Build history of the part. All positions in model axes, mm. A direction names the side the tool comes from. Round coordinates to 2 decimals unless told otherwise and drop trailing zeros. Write each loop counter-clockwise with the first axis right and the second up, starting at its lowest first coordinate (ties: lowest second). Pieces come first, ordered by that corner, then holes. Notation, with made-up numbers: M 80,49 L 124,49 A21 ccw 124,72 Z; hole C 65.25,48.25 d5. An arc over 180 degrees is marked long. Write item = value, one per line. Start each with the question number.
Q1. Drop flat-ended pins along their axis: P1, Ø4, axis at y = -22.5, z = 5, coming from the -X side; P2, Ø10, axis at x = -8.5, y = 9.5, coming from the +Z side; P3, Ø1.5, axis at x = -44.5, z = 13, coming from the +Y side; P4, Ø2.5, axis at y = 24.5, z = 13, coming from the +X side. Give the stop position or say it passes through.
Q2. Band-saw the part on A-A on x = 51. Write the cut outline in (y, z), plus the area to 3 significant figures.
Q3. Pull direction Y, two halves, no side cores. Call faces 5 (the flat face through (0, 18, 0)), 6 (the flat face through (0, 33.092, 7)), 7 (the flat face through (0, 34.092, 13)): released by +Y, released by -Y, zero draft, split by the parting line, or undercut.
Q4. Probe L1, parallel to X at y = 24, z = 14; L2, parallel to Y at x = -74.5, z = 6.25; L3, parallel to Y at x = -62.5, z = 10.5. List the from-to ranges inside material, lowest first.
Q5. Band-saw the part on D-D on z = 12.25. Write the cut outline in (x, y).
Q6. Band-saw the part on B-B on y = -47. Write the cut outline in (x, z), plus the area to 3 significant figures.
Q7. Tool access for faces 1 (the flat face through (-83.74, -12, 13)), 2 (the flat face through (2, -54.908, 10)), 3 (the flat face through (1, -56, 5.762)), 4 (the flat face through (-82.74, -2, 9)): list every direction of +Z, -Z, +X, -X, +Y, -Y with a clear straight run to the whole face (end or side of a thin tool).
Q8. Band-saw the part on C-C on x = 16. Write the cut outline in (y, z), plus the area to 3 significant figures.
```python
from build123d import *

# Parameters (mm, degrees)
SKETCH_1_W               = 172
SKETCH_1_H               = 92
EXTRUDE_1_DEPTH          = 2
SKETCH_2_W               = 32
SKETCH_2_H               = 22
CUT_EXTRUDE_1_DEPTH      = 2
SKETCH_3_R               = 6.5
CUT_EXTRUDE_2_DEPTH      = 2
SKETCH_4_W               = 172
SKETCH_4_H               = 92
EXTRUDE_3_DEPTH          = 13
SKETCH_5_W               = 168
SKETCH_5_H               = 55.87
CUT_EXTRUDE_3_DEPTH      = 18
CUT_EXTRUDE_4_DEPTH      = 182.789670088
CUT_EXTRUDE_4_DEPTH_BACK = 172
FILLET_1_R               = 15
SKETCH_7_W               = 10
SKETCH_7_H               = 10
CUT_EXTRUDE_5_DEPTH      = 2
CUT_EXTRUDE_6_DEPTH      = 5
FILLET_2_R               = 2
FILLET_3_R               = 1.5


with BuildPart() as part:
    # 草图1 → 凸台-拉伸1 (new body)
    with BuildSketch(Plane.XY):
        with Locations((1.259970458, -10.907680945)):
            Rectangle(SKETCH_1_W, SKETCH_1_H)
    extrude(amount=EXTRUDE_1_DEPTH)

    # 草图2 → 切除-拉伸1 (cut)
    with BuildSketch(Plane(origin=(0, 0, 0), x_dir=(-1, 0, 0), z_dir=(0, 0, -1))):
        with Locations((-60.259970458, 22.092319055)):
            Rectangle(SKETCH_2_W, SKETCH_2_H)
    extrude(amount=-CUT_EXTRUDE_1_DEPTH, mode=Mode.SUBTRACT)

    # 草图3 → 切除-拉伸2 (cut)
    with BuildSketch(Plane(origin=(0, 0, 0), x_dir=(-1, 0, 0), z_dir=(0, 0, -1))):
        with Locations((54.740029542, 24.092319055)):
            Circle(SKETCH_3_R)
        with Locations((71.740029542, 25.092319055)):
            Circle(SKETCH_3_R)
    extrude(amount=-CUT_EXTRUDE_2_DEPTH, mode=Mode.SUBTRACT)

    # 草图4 → 凸台-拉伸3 (add)
    with BuildSketch(Plane.XY.offset(2)):
        with Locations((1.259970458, -10.907680945)):
            Rectangle(SKETCH_4_W, SKETCH_4_H)
        Polygon((-82.740029542, -54.907680945), (-82.740029542, 33.092319055), (44.259970458, 33.092319055), (76.259970458, 33.092319055), (85.259970458, 33.092319055), (85.259970458, -54.907680945), align=None, mode=Mode.SUBTRACT)
    extrude(amount=EXTRUDE_3_DEPTH)

    # 草图5 → 切除-拉伸3 (cut)
    with BuildSketch(Plane(origin=(0, 0, 0), x_dir=(-1, 0, 0), z_dir=(0, 0, -1))):
        with Locations((-1.259970458, -26.972680945)):
            Rectangle(SKETCH_5_W, SKETCH_5_H)
    extrude(amount=-CUT_EXTRUDE_3_DEPTH, mode=Mode.SUBTRACT)

    # 草图6 → 切除-拉伸4 (cut, two sides: drawn at the far end of the back side and taken through both)
    with BuildSketch(Plane(origin=(87.259970458, 0, 0), x_dir=(0, 0, -1), z_dir=(1, 0, 0)).offset(-CUT_EXTRUDE_4_DEPTH_BACK)):
        Polygon((84.64151075, 176.551763032), (0, 0.962319055), (-5.76238744, -10.991796575), (-5.76238744, -56.907680945), (-5.76238744, -251.832892702), (375.68654555, -332.33173887), (466.09044374, 96.052916865), align=None)
    extrude(amount=CUT_EXTRUDE_4_DEPTH + CUT_EXTRUDE_4_DEPTH_BACK, mode=Mode.SUBTRACT)

    # 圆角1
    fillet_1_edges = [part.edges().sort_by_distance(p)[0] for p in [
        (86.259970458, -10.991796575, 5.76238744),
        (-83.740029542, -10.991796575, 5.76238744),
    ]]
    fillet(fillet_1_edges, radius=FILLET_1_R)

    # 草图7 → 切除-拉伸5 (cut)
    with BuildSketch(Plane(origin=(87.259970458, 0, 0), x_dir=(0, 0, -1), z_dir=(1, 0, 0))):
        with Locations((-10, 12.092319055)):
            Rectangle(SKETCH_7_W, SKETCH_7_H)
    extrude(amount=-CUT_EXTRUDE_5_DEPTH, mode=Mode.SUBTRACT)

    # 草图8 → 切除-拉伸6 (cut)
    with BuildSketch(Plane.XY.offset(15)):
        Polygon((-83.740029542, -55.907680945), (-83.740029542, 34.092319055), (86.259970458, 34.092319055), (86.259970458, 17.092319055), (87.259970458, 17.092319055), (87.259970458, 35.092319055), (-84.740029542, 35.092319055), (-84.740029542, -56.907680945), (87.259970458, -56.907680945), (87.259970458, 7.092319055), (86.259970458, 7.092319055), (86.259970458, -55.907680945), align=None)
    extrude(amount=-CUT_EXTRUDE_6_DEPTH, mode=Mode.SUBTRACT)

    # 圆角2
    fillet_2_edges = [part.edges().sort_by_distance(p)[0] for p in [
        (76.259970458, 11.092319055, 1),
        (76.259970458, 33.092319055, 1),
        (44.259970458, 33.092319055, 1),
        (44.259970458, 11.092319055, 1),
    ]]
    fillet(fillet_2_edges, radius=FILLET_2_R)

    # 圆角3
    fillet_3_edges = [part.edges().sort_by_distance(p)[0] for p in [
        (-84.740029542, 35.092319055, 5),
        (87.259970458, 35.092319055, 5),
        (87.259970458, -56.907680945, 7.88119372),
        (-84.740029542, -56.907680945, 7.88119372),
        (1.259970458, 35.092319055, 0),
        (-84.740029542, 18.027319055, 0),
        (87.259970458, 18.027319055, 0),
    ]]
    fillet(fillet_3_edges, radius=FILLET_3_R)


solid = part.part
```
Conclusion:
q1.P1 = -84.74
q1.P2 = 2
q1.P3 = 34.09
q1.P4 = 86.26
q2.outline = M -56.91,5.76 L -54.91,5.76 L -54.91,15 L -55.91,15 L -55.91,10 L -56.91,10 Z; M 0.96,0 L 11.09,0 L 11.09,2 L 0.96,2 Z; M 33.09,0 L 33.59,0 A1.5 ccw 35.09,1.5 L 35.09,10 L 34.09,10 L 34.09,15 L 33.09,15 Z
q2.area = 58.3 mm^2
q3.face_5 = zero draft
q3.face_6 = undercut
q3.face_7 = released by +Y
q4.L1 = -83.74 to -82.74, 85.26 to 86.26
q4.L2 = -56.91 to -54.91, 33.09 to 35.09
q4.L3 = -55.91 to -54.91, 33.09 to 34.09
q5.outline = M -83.74,-55.91 L 86.26,-55.91 L 86.26,7.09 L 85.26,7.09 L 85.26,-54.91 L -82.74,-54.91 L -82.74,33.09 L 85.26,33.09 L 85.26,17.09 L 86.26,17.09 L 86.26,34.09 L -83.74,34.09 Z
q6.outline = M -84.74,5.76 L -82.74,5.76 L -82.74,15 L -83.74,15 L -83.74,10 L -84.74,10 Z; M 85.26,5.76 L 87.26,5.76 L 87.26,10 L 86.26,10 L 86.26,15 L 85.26,15 Z
q6.area = 27.0 mm^2
q7.face_1 = +Z, -X, +Y, -Y
q7.face_2 = +Z, -Z
q7.face_3 = -Z, +X, -X, -Y
q7.face_4 = +Z
q8.outline = M -56.91,5.76 L -54.91,5.76 L -54.91,15 L -55.91,15 L -55.91,10 L -56.91,10 Z; M 0.96,0 L 33.59,0 A1.5 ccw 35.09,1.5 L 35.09,10 L 34.09,10 L 34.09,15 L 33.09,15 L 33.09,2 L 0.96,2 Z
q8.area = 102 mm^2
